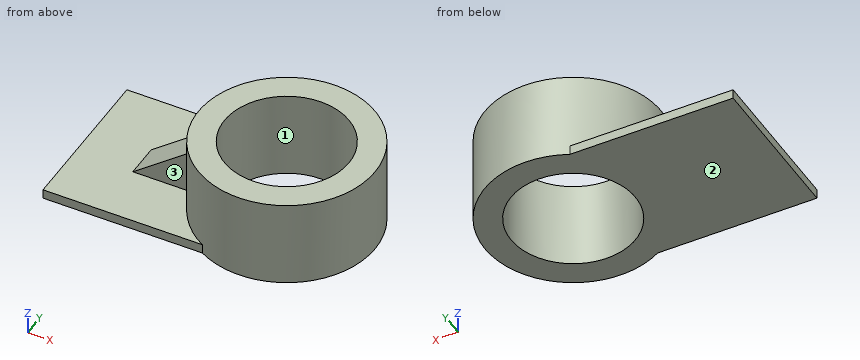
```python
from build123d import *

# Parameters (mm, degrees)
F0_R     = 37.539526
F1_DEPTH = 37.592
F2_W     = 69.573917
F2_H     = 66.385109
F3_DEPTH = 4.064
F4_R     = 26.450097
F5_DEPTH = 37.593
F7_DEPTH = 19.05
F9_DEPTH = 45.0777


with BuildPart() as f1:
    # F0 (on Top) → F1 (new body)
    with BuildSketch(Plane.XY):
        with Locations((21.162063, 0)):
            Circle(F0_R)
    extrude(amount=F1_DEPTH)

    # F2 (on Top) → F3 (join)
    with BuildSketch(Plane.XY):
        with Locations((-30.148695, 0.434836)):
            Rectangle(F2_W, F2_H)
    extrude(amount=F3_DEPTH)

    # F4 (on face) → F5 (cut, through all)
    with BuildSketch(Plane.XY.offset(37.592)):
        with Locations((21.162063, 0)):
            Circle(F4_R)
    extrude(amount=-F5_DEPTH, mode=Mode.SUBTRACT)

    # F6 (on face) → F7 (join)
    with BuildSketch(Plane.XY.offset(4.064)):
        with BuildLine():
            ThreePointArc((-15.713447, -7.029422), (-16.377463, 0), (-15.713447, 7.029422))
            Line((-15.713447, 7.029422), (-40.294893, 7.029422))
            Line((-40.294893, 7.029422), (-40.294893, -7.537174))
            Line((-40.294893, -7.537174), (-15.713447, -7.537174))
            Line((-15.713447, -7.537174), (-15.713447, -7.029422))
        make_face()
    extrude(amount=F7_DEPTH)

    # F8 (on face) → F9 (cut, through all)
    with BuildSketch(Plane.XZ.offset(7.537174)):
        Polygon((-40.294893, 23.114), (-40.294893, 4.064), (-15.713447, 23.114), align=None)
    extrude(amount=-F9_DEPTH, mode=Mode.SUBTRACT)


solid = f1.part
```
Here's how the part is built. I have some questions about the finished solid (model axes, mm). Face numbers are marked on the shaded views. Round coordinates to 2 decimals unless told otherwise and drop trailing zeros. Write each loop counter-clockwise with the first axis right and the second up, starting at its lowest first coordinate (ties: lowest second). Pieces come first, ordered by that corner, then holes.
Q1. Will these pins go through, and if not, where does the flat tip stop? P1, Ø1.2, axis at x = -34, z = 1.5, coming from the +Y side; P2, Ø12, axis at y = -15.5, z = 15, coming from the +X side; P3, Ø21, axis at x = -31.5, z = 16.5, coming from the -Y side.
Q2. If we section it at A-A on y = 0: Write out the boundary of the cut face in (x, z), plus the area to 3 significant figures.
Q3. If we section it at D-D on x = -9.5: Write out the boundary of the cut face in (y, z), plus the area to 3 significant figures.
Q4. If we mould it in two halves opening along Y, with no side actions, what happens to the marked faces 1, 2 and 3? For each: +Y half, -Y half, draft (parallel to the pull), parting line (faces both ways), or undercut.
Q5. If we section it at C-C on z = 28: Write out the boundary of the cut face in (x, y), plus the area to 3 significant figures.
Q6. If we section it at B-B on x = 10: Write out the boundary of the cut face in (y, z).
Q7. Please list where these lines run through material, in increasing order: probe 1 along X at (y, z) = (0.5, 27); probe 2 along Y at (x, z) = (-31, 8); probe 3 along Z at (x, y) = (-58.5, -11.5).
Answer below:
1. P1: stops at y = 33.63
1. P2: stops at x = 57.48
1. P3: stops at y = -7.54
2. outline: (-64.94, 0) - (-5.29, 0) - (-5.29, 37.59) - (-16.38, 37.59) - (-16.38, 23.11) - (-15.71, 23.11) - (-40.29, 4.06) - (-64.94, 4.06) - close; (47.61, 0) - (58.7, 0) - (58.7, 37.59) - (47.61, 37.59) - close
2. area: 1,250 mm2
3. outline: (-32.76, 0) - (33.63, 0) - (33.63, 4.06) - (21.66, 4.06) - (21.66, 37.59) - (-21.66, 37.59) - (-21.66, 4.06) - (-32.76, 4.06) - close
3. area: 1,720 mm2
4. face 1: undercut
4. face 2: draft
4. face 3: -Y half
5. outline: circle Ø75.08 at (21.16, 0); hole circle Ø52.9 at (21.16, 0)
5. area: 2,230 mm2
6. outline: (-35.84, 0) - (-23.98, 0) - (-23.98, 37.59) - (-35.84, 37.59) - close; (23.98, 0) - (35.84, 0) - (35.84, 37.59) - (23.98, 37.59) - close
7. probe 1: x = -16.37 to -5.28, 47.61 to 58.7
7. probe 2: y = -7.54 to 7.03
7. probe 3: z = 0 to 4.06
